Autodesk Inventor part; units mm, degrees
ref_plane "YZ Plane" through (0, 0, 0) normal (1, 0, 0) x (0, 1, 0)
ref_plane "XZ Plane" through (0, 0, 0) normal (0, 1, 0) x (-1, 0, 0)
ref_plane "XY Plane" through (0, 0, 0) normal (0, 0, 1) x (1, 0, 0)
sketch "Эскиз1" plane through (0, 0, 0) normal (0, 1, 0) x (-1, 0, 0)
  circle A0 centre (0, 0) radius 56
  dimension "d0" = 112
extrude "Выдавливание1" add sketch "Эскиз1" along normal blind 10
sketch "Эскиз2" plane through (0, 10, 0) normal (0, 1, 0) x (1, 0, 0)
  circle A0 centre (0, 0) radius 38
  dimension "d3" = 76
extrude "Выдавливание2" add sketch "Эскиз2" along normal blind 38
sketch "Эскиз3" plane through (0, 10, 0) normal (0, 1, 0) x (1, 0, 0)
  point P0 (0, 0)
  point P1 (-46, 0)
  dimension "d8" = 46
hole "Отверстие1" at (-46, 10, 0) direction (0, -1, 0) diameter 11 end through all
pattern_circular "Круговой массив1" count 4 over 360 about axis through (0, -10, 0) along (0, 1, 0) of "Отверстие1"
sketch "Эскиз4" plane through (0, 0, 0) normal (0, -1, 0) x (1, 0, 0)
  circle A0 centre (0, 0) radius 22
  dimension "d19" = 44
extrude "Выдавливание3" cut sketch "Эскиз4" against normal blind 10
sketch "Эскиз5" plane through (0, 48, 0) normal (0, 1, 0) x (1, 0, 0)
  circle A0 centre (0, 0) radius 12.5
  dimension "d22" = 25
extrude "Выдавливание4" cut sketch "Эскиз5" against normal through all
fillet "Сопряжение1" radius 2 1 edges at (-38, 10, 0)
chamfer "Фаска1" distance 1.6 angle 45 1 edges at (-22, 0, 0)
chamfer "Фаска2" distance 2.5 angle 45 1 edges at (-38, 48, 0)
sketch "Эскиз6" plane through (0, 48, 0) normal (0, 1, 0) x (1, 0, 0)
  point P0 (0, 0)
  point P1 (-24, 0)
  point P2 (24, 0)
  dimension "d32" = 24
  dimension "d33" = 48
hole "Отверстие2" at (-24, 48, 0) at (24, 48, 0) direction (0, -1, 0) diameter 8.376 depth 29 tip angle 120
chamfer "Фаска3" distance 1.6 angle 45 2 edges at (-24, 48, -4.188) (24, 48, -4.188)
properties part number "Фланецц"
Work out the finished part from the listing and answer in its coordinate system (mm). A direction names the side the tool comes from. Give positions to 0.01 mm unless a question says otherwise; leave off trailing zeros. Loops run counter-clockwise (first coordinate to the right, second up) from the corner with the lowest first, then second, coordinate; pieces in that order, holes last. Notation, with made-up numbers: (5, -2) -> (42, -2) arc R31 cw to (42, 27) -> close; hole circle Ø11 at (-37, 38.25). An arc over 180 degrees is marked (long way). Use CSV: the item, a comma, the result in double quotes.
1. Straight lines are drawn through the part: line 1 (Z direction, x = 0, y = 5); line 2 (X direction, y = 39.5, z = 0); line 3 (Y direction, x = 14.5, z = -3.5). For each, find the intervals that lie inside material, in ascending order.
Found:
line 1,"-56 to -51.5, -40.5 to -22, 22 to 40.5, 51.5 to 56"
line 2,"-38 to -28.19, -19.81 to -12.5, 12.5 to 19.81, 28.19 to 38"
line 3,"10 to 48"
2. The part is cut by section D-D (y = 44). Write down the section's boundary in (x, z).
Found:
outline,"circle Ø76 at (0, 0); hole circle Ø8.38 at (-24, 0); hole circle Ø25 at (0, 0); hole circle Ø8.38 at (24, 0)"
3. The part is cut by section A-A (x = 0). State how many separate pieces and enclosed holes the cut face has, then the cut area to 3 significant figures.
Found:
separate pieces,"4"
enclosed holes,"0"
area,"2,390 mm^2"
4. The mould has two halves that part along X. Classify faces 4 (the flat face through (1, 0, -24)), 5 (the cylindrical face through (-51.73, 4.93, 21.45)), 6 (the cylindrical face through (-0.716, 4.93, 51.453)): +X half, -X half, draft (parallel to the pull), parting line (faces both ways), or undercut.
Found:
face 4,"draft"
face 5,"parting line"
face 6,"undercut"
5. The part is cut by section B-B (z = 43). Write down the section's boundary in (x, y), then the cut area to 3 significant figures.
Found:
outline,"(-35.87, 0) -> (-4.61, 0) -> (-4.61, 10) -> (-35.87, 10) -> close; (4.61, 0) -> (35.87, 0) -> (35.87, 10) -> (4.61, 10) -> close"
area,"625 mm^2"
6. The part is cut by section C-C (x = 43). Write down the section's boundary in (y, z).
Found:
outline,"(0, -35.87) -> (10, -35.87) -> (10, -4.61) -> (0, -4.61) -> close; (0, 4.61) -> (10, 4.61) -> (10, 35.87) -> (0, 35.87) -> close"
7. A tool of negligible diameter and unlimited length cuts with its end or side. For faces 1 (the flat face through (0, 48, 15)), 2 (the cylindrical face through (-4.769, 5.741, -21.477)), 3 (the cylindrical face through (17.535, 28.516, -33.713)), from which of +Z, -Z, +X, -X, +Y, -Y can it reach the whole face along a straight path? Write none if from no direction.
Found:
face 1,"+Z, -Z, +X, -X, +Y"
face 2,"-Y"
face 3,"+Y"
8. Flat-ended cylindrical pins translate along their axes: pin 1 Ø4 at (y, z) = (25, -9.5) entering from +X; pin 2 Ø6.5 at (x, z) = (24, 0) entering from -Y; pin 3 Ø10 at (x, y) = (8.5, 26.5) entering from +Z; pin 4 Ø22 at (x, z) = (-11, 5) entering from -Y. Find the tip coordinate at first contact, or state that the pin passes through.
Found:
pin 1,"x = 37.25"
pin 2,"y = 0"
pin 3,"z = 37.84"
pin 4,"y = 0.52"
